Autodesk Inventor part; units mm, degrees
ref_plane "YZ Plane" through (0, 0, 0) normal (1, 0, 0) x (0, 1, 0)
ref_plane "XZ Plane" through (0, 0, 0) normal (0, 1, 0) x (-1, 0, 0)
ref_plane "XY Plane" through (0, 0, 0) normal (0, 0, 1) x (1, 0, 0)
sketch "Sketch1" plane through (0, 0, 0) normal (0, 0, 1) x (1, 0, 0)
  line L0 (0, 0) -> (0, 1550)
  line L1 (0, 1550) -> (-168.8166, 1550)
  line L2 (-168.8166, 1550) -> (-194.9992, 50)
  line L3 (-194.9992, 50) -> (-194.9992, 0) construction
  line L4 (-194.9992, 0) -> (0, 0)
  line L5 (-169.6893, 1500.0076) -> (-174.6885, 1500.0949)
  line L6 (-174.6885, 1500.0949) -> (-200, 50)
  line L7 (-200, 50) -> (-200, 0)
  line L8 (-200, 0) -> (-194.9992, 0)
  line L9 (-200, 50) -> (-194.9992, 50) construction
  dimension "d0" = 1550
  dimension "d1" = 168.8166
  dimension "d2" = 5
  dimension "d3" = 200
  dimension "d4" = 50
  dimension "d6" = 50
  dimension "d17" = 89
extrude "Plate1" add sketch "Sketch1" along normal blind 3.048
sketch "Sketch2" plane through (-3.048, 0, 3.048) normal (1, 0, 0) x (0, 1, 0)
  line L0 (1550, 0) -> (0, 0)
  line L1 (0, 0) -> (0, -28)
  line L2 (0, -28) -> (1550, -28)
  line L3 (1550, -28) -> (1550, 0)
edge flange "Flange1" height 28 angle 90 thickness 3.048 bend radius 3.048 thickness toward (1, 0, 0) relief tear relief width 3.048 relief depth 1.524 edges at (0, 775, 0) wall of the first edge with corners at (-3.048, 1550, 3.048) (-3.048, 0, 3.048) (-3.048, 0, -24.952) (-3.048, 1550, -24.952)
bend "Bend1"
corner "Corner1"
equation "\"d5\" = Thickness"
equation "\"d7\" = BendReliefWidth"
equation "\"d8\" = BendReliefDepth"
equation "\"d9\" = MinimumRemnant"
equation "\"d10\" = TransitionRadius"
equation "\"d13\" = BendRadius"
equation "\"d14\" = CornerReliefSize"
equation "\"d15\" = GapSize"
equation "\"d16\" = JacobiRadiusSize"
equation "\"BendRadius\" = Thickness"
equation "\"BendReliefWidth\" = Thickness"
equation "\"BendReliefDepth\" = 0.5 * Thickness"
equation "\"CornerReliefSize\" = 4 * Thickness"
equation "\"MinimumRemnant\" = 2 * Thickness"
equation "\"TransitionRadius\" = BendRadius"
equation "\"JacobiRadiusSize\" = BendRadius"
equation "\"GapSize\" = Thickness"
Check sheet for the modelled part. Datum: model origin and axes. Units: mm. A direction names the side the tool comes from. Give positions to 0.01 mm unless a question says otherwise; leave off trailing zeros. Write each loop counter-clockwise with the first axis right and the second up, starting at its lowest first coordinate (ties: lowest second). Pieces come first, ordered by that corner, then holes.
Item 1: Scan lines: L1, parallel to Z at x = -72, y = 1385.5; L2, parallel to X at y = 1276, z = -19.75; L3, parallel to X at y = 1392, z = -2.5. Record each from-to range of solid material in increasing order.
Item 2: Cross-section at B-B (x = -52). Enter the section's corners in (y, z).
Item 3: Cross-section at C-C (z = -12.5). Enter the section's corners in (x, y).
Item 4: Access from +Z, -Z, +X, -X, +Y, -Y to the whole of each face (thin tool, end or side, straight path). Record for faces 1 (the face through (-104, 786, 3.048)), 2 (the face through (-104, 786, 0)).
Item 5: Gauge pin test, flat ends, axial feed: pin 1 (6 mm diameter, centred on x = -39.5, y = 330.5, fed in from -Z); pin 2 (6 mm diameter, centred on y = 1283.5, z = -0.5, fed in from -X); pin 3 (6.5 mm diameter, centred on y = 524, z = -19, fed in from -X). Record the tip position at first contact, or that the pin passes through.
Item 6: Cross-section at A-A (y = 1320.5). Enter the section's corners in (x, z).
Item 7: Cross-section at D-D (y = 1074). Enter the section's corners in (x, z), and give its area (3 significant figures).
Report:
1. L1: z = 0 to 3.05
1. L2: x = -3.05 to 0
1. L3: x = -3.1 to -0.02
2. outline: (0, 0) - (1550, 0) - (1550, 3.05) - (0, 3.05) - close
3. outline: (-3.05, 0) - (0, 0) - (0, 1550) - (-3.05, 1550) - close
4. face 1: +Z, +X, -X, +Y, -Y
4. face 2: -Z, -X, +Y, -Y
5. pin 1: stops at z = 0
5. pin 2: stops at x = -178.52
5. pin 3: stops at x = -3.05
6. outline: (-177.82, 0) - (-6.1, 0) arc R3.05 cw to (-3.05, -3.05) - (-3.05, -24.95) - (0, -24.95) - (0, -3.05) arc R6.1 ccw to (-6.1, 3.05) - (-177.82, 3.05) - close
7. outline: (-182.13, 0) - (-6.1, 0) arc R3.05 cw to (-3.05, -3.05) - (-3.05, -24.95) - (0, -24.95) - (0, -3.05) arc R6.1 ccw to (-6.1, 3.05) - (-182.13, 3.05) - close
7. area: 625 mm2
